Check sheet for the drawn part. Datum: minimum x, y, z corner. Units: mm. A direction names the side the tool comes from. Coordinates: 2 decimals unless noted, no trailing zeros. Order: outer loops, then holes, each group sorted by start corner. A loop starts at its lowest first (then second) coordinate and runs counter-clockwise, first axis right, second up.
1. Set-up check for the marked faces 1 and 2: record each of +Z, -Z, +X, -X, +Y, -Y from which the full face is reachable in a straight line by a thin tool's end or side.
2. Cross-section at C-C (y = 8.5). Enter the section's corners in (x, z), then the cut area to 3 significant figures.
3. Cross-section at A-A (y = 14). Enter the section's corners in (x, z), then the cut area to 3 significant figures.
4. Draft check along Z on the marked faces 3 and 4. Enter one of: released by +Z, released by -Z, zero draft, split by the parting line, or undercut.
5. Gauge pin test, flat ends, axial feed: pin 1 Ø4 at (x, z) = (7.14, 13) entering from -Y; pin 2 Ø4 at (y, z) = (1.5, 14.5) entering from -X; pin 3 Ø6 at (y, z) = (14, 37.5) entering from +X (1 decimal); pin 4 Ø4 at (x, y) = (24.5, 10.5) entering from +Z. Record the tip position at first contact, or that the pin passes through.
6. Thickness scan on line 1 (Z direction, x = 21, y = 1.4); line 2 (Y direction, x = 14, z = 38); line 3 (Z direction, x = 37, y = 14) (1 decimal). Record the ranges inside material, lowest first.
7. Cross-section at B-B (x = 21). Count the separate pieces of the cut face and the enclosed holes in it, then the cut area to 3 significant figures.
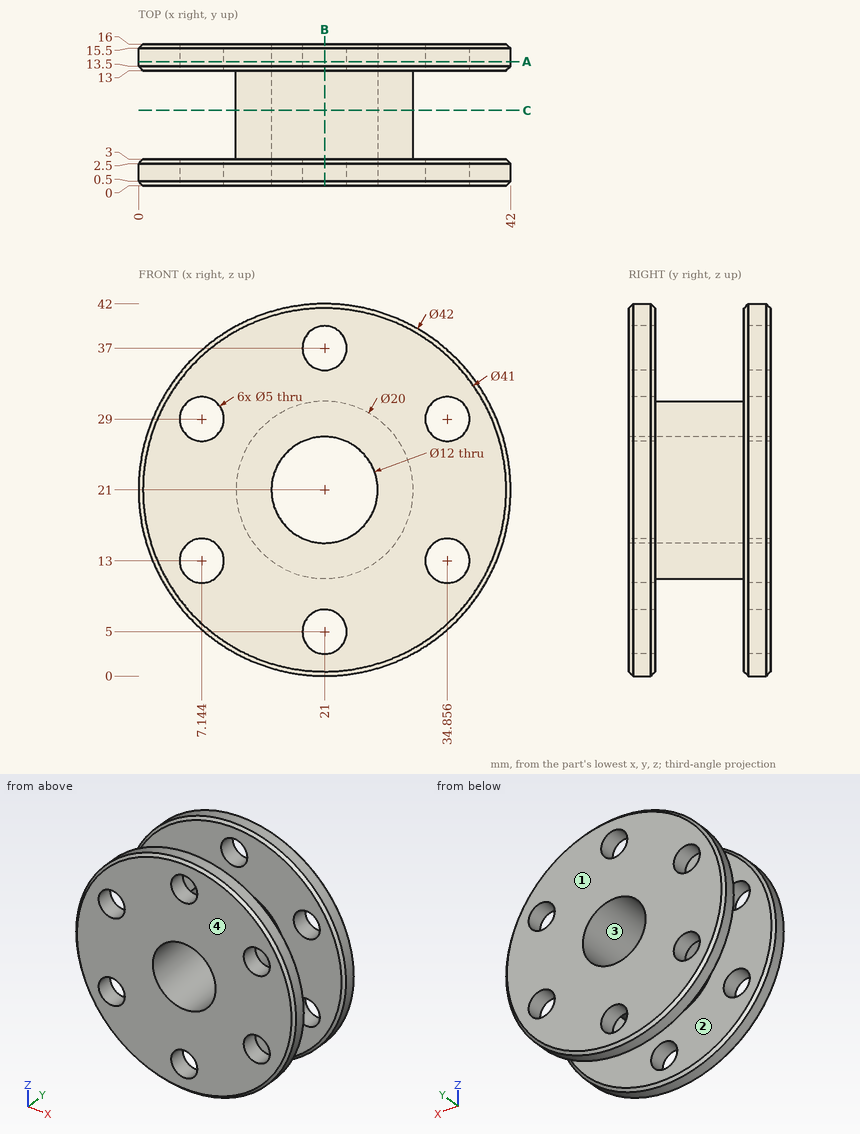
Data:
1. face 1: +Z, -Z, +X, -X, +Y
1. face 2: none
2. outline: circle Ø20 at (21, 21); hole circle Ø12 at (21, 21)
2. area: 201 mm2
3. outline: circle Ø42 at (21, 21); hole circle Ø5 at (7.14, 13); hole circle Ø5 at (7.14, 29); hole circle Ø12 at (21, 21); hole circle Ø5 at (21, 5); hole circle Ø5 at (21, 37); hole circle Ø5 at (34.86, 13); hole circle Ø5 at (34.86, 29)
3. area: 1,150 mm2
4. face 3: undercut
4. face 4: zero draft
5. pin 1: passes through
5. pin 2: stops at x = 0.49
5. pin 3: stops at x = 37.1
5. pin 4: stops at z = 30.89
6. line 1: z = 0 to 2.5, 7.5 to 15, 27 to 34.5, 39.5 to 42
6. line 2: y = 0 to 3, 13 to 16
6. line 3: z = 7.4 to 11.7, 14.3 to 27.7, 30.3 to 34.6
7. separate pieces: 6
7. enclosed holes: 0
7. area: 199 mm2
